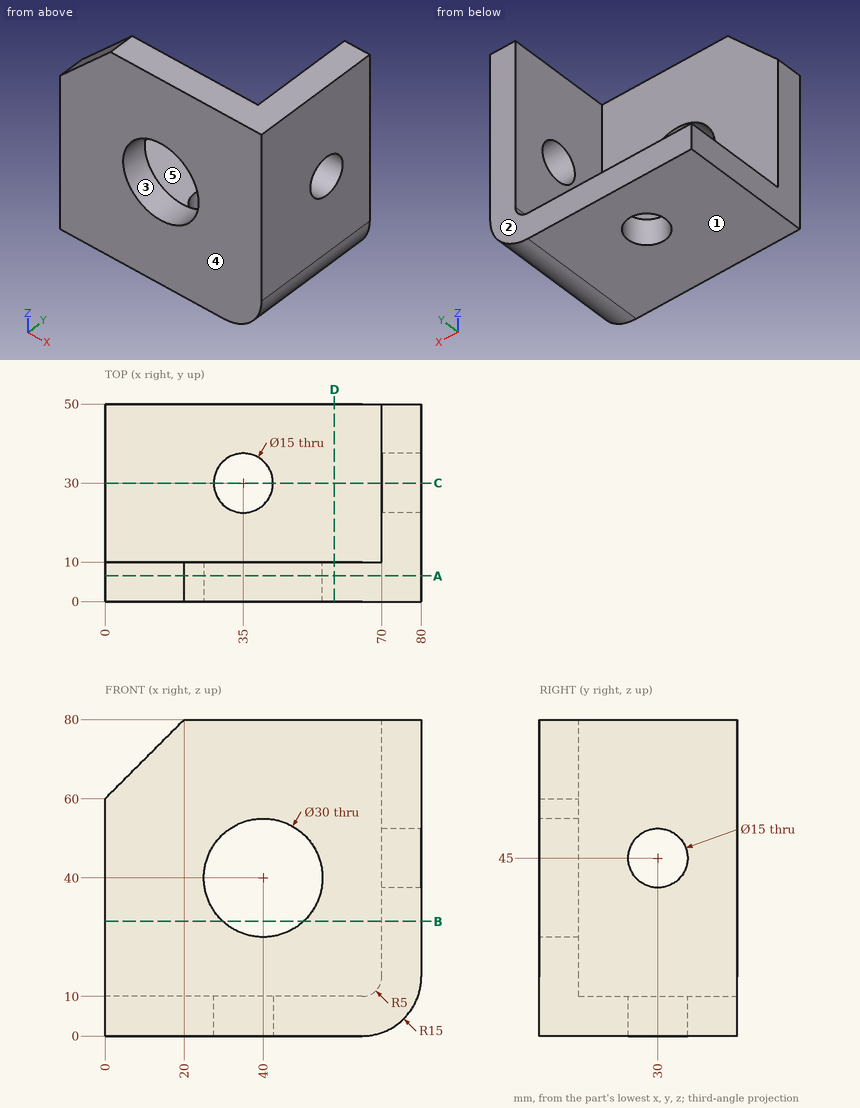
Here's the drawing with two shaded views (mm, measured from the low corner). I have some questions. A direction names the side the tool comes from. Coordinates: 2 decimals unless noted, no trailing zeros. Loops run counter-clockwise (first coordinate to the right, second up) from the corner with the lowest first, then second, coordinate; pieces in that order, holes last.
Item 1: I'm going to push flat-ended pins straight in: pin 1 (10 mm diameter, centred on y = 34, z = 26, fed in from -X); pin 2 (13.5 mm diameter, centred on x = 35, y = 30, fed in from -Z); pin 3 (21 mm diameter, centred on x = 27.5, z = 57.5, fed in from +Y); pin 4 (20 mm diameter, centred on x = 44, y = 21.5, fed in from +Z). Where does each tip first touch, or does it pass through?
Answers below:
pin 1: stops at x = 70
pin 2: passes through
pin 3: stops at y = 10
pin 4: stops at z = 10
Item 2: If we mould it in two halves opening along Z, with no side actions, what happens to the marked faces 1, 2 and 3? For each: released by +Z, released by -Z, zero draft, split by the parting line, or undercut.
Answers below:
face 1: released by -Z
face 2: zero draft
face 3: undercut
Item 3: Suppose I cut it at A-A (y = 6.5). Please give me the cut outline in (x, z).
Answers below:
outline: (0, 0) - (65, 0) arc R15 ccw to (80, 15) - (80, 80) - (20, 80) - (0, 60) - close; hole circle Ø30 at (40, 40)
Item 4: Suppose I cut it at D-D (x = 58). Please give me the cut outline in (y, z), then the cut area to 3 significant figures.
Answers below:
outline: (0, 0) - (50, 0) - (50, 10) - (10, 10) - (10, 80) - (0, 80) - close
area: 1,200 mm2
Item 5: Which directions (+Z, -Z, +X, -X, +Y, -Y) give clear straight access to the entire face, cutting with the end or side of a thin tool? Please do the marked faces 4 and 5.
Answers below:
face 4: +Z, -Z, +X, -X, -Y
face 5: +Z, -X, +Y
Item 6: Suppose I cut it at B-B (z = 29). Please give me the cut outline in (x, y), then the cut area to 3 significant figures.
Answers below:
outline: (0, 0) - (29.8, 0) - (29.8, 10) - (0, 10) - close; (50.2, 0) - (80, 0) - (80, 50) - (70, 50) - (70, 10) - (50.2, 10) - close
area: 996 mm2
Item 7: Suppose I cut it at C-C (y = 30). Please give me the cut outline in (x, z).
Answers below:
outline: (0, 0) - (27.5, 0) - (27.5, 10) - (0, 10) - close; (42.5, 0) - (65, 0) arc R15 ccw to (80, 15) - (80, 37.5) - (70, 37.5) - (70, 15) arc R5 cw to (65, 10) - (42.5, 10) - close; (70, 52.5) - (80, 52.5) - (80, 80) - (70, 80) - close
Item 8: Please list where these lines run through material, in increasing order: L1, parallel to X at y = 5.5, z = 40; L2, parallel to X at y = 39.5, z = 15.5.
Answers below:
L1: x = 0 to 25, 55 to 80
L2: x = 70 to 80
